from build123d import *

# Parameters (mm, degrees)
F0_R            = 56
F0_R_2          = 62.5
F1_DEPTH        = 35
F3_DEPTH        = 1
F4_W            = 26
F4_H            = 35
F5_DEPTH        = 50
F6_W            = 8
F6_H            = 10
F7_DEPTH        = 26
F8_R            = 17.5
F9_DEPTH        = 50
F10_R           = 2
F12_D           = 3
F12_DEPTH       = 8
F12_CBORE_D     = 5
F12_CBORE_DEPTH = 2
F14_D           = 3
F14_DEPTH       = 8
F14_CBORE_D     = 5
F14_CBORE_DEPTH = 2


with BuildPart() as f1:
    # F0 (on Top) → F1 (new body)
    with BuildSketch(Plane.XY):
        with Locations((-62.5, 0)):
            Circle(F0_R)
        with Locations((-62.5, 0)):
            Circle(F0_R_2)
        with Locations((-62.5, 0)):
            Circle(F0_R, mode=Mode.SUBTRACT)
    extrude(amount=F1_DEPTH)

    # F2 (on Right) → F3 (join)
    with BuildSketch(Plane.YZ):
        Polygon((-13, 0), (0, 0), (13, 0), (13, 35), (-13, 35), align=None)
    extrude(amount=-F3_DEPTH)

    # F4 (on face) → F5 (join)
    with BuildSketch(Plane.YZ):
        with Locations((0, 17.5)):
            Rectangle(F4_W, F4_H)
    extrude(amount=F5_DEPTH)

    # F6 (on face) → F7 (join)
    with BuildSketch(Plane.XZ.offset(13)):
        with Locations((42, 40)):
            Rectangle(F6_W, F6_H)
        with Locations((12, 40)):
            Rectangle(F6_W, F6_H)
    extrude(amount=-F7_DEPTH)

    # F8 (on face) → F9 (cut)
    with BuildSketch(Plane.XZ.offset(13)):
        with Locations((27, 21.5)):
            Circle(F8_R)
    extrude(amount=-F9_DEPTH, mode=Mode.SUBTRACT)

    # F10
    f10_edges = [f1.edges().sort_by_distance(p)[0] for p in [
        (46, 0, 35),
        (8, 0, 35),
    ]]
    fillet(f10_edges, radius=F10_R)

    # F12
    with Locations(Plane.YZ.offset(46)):
        with Locations((0, 41)):
            CounterBoreHole(F12_D / 2, F12_CBORE_D / 2, F12_CBORE_DEPTH, depth=F12_DEPTH)

    # F14
    with Locations(Plane(origin=(8, 0, 0), x_dir=(0, -1, 0), z_dir=(-1, 0, 0))):
        with Locations((0, 41)):
            CounterBoreHole(F14_D / 2, F14_CBORE_D / 2, F14_CBORE_DEPTH, depth=F14_DEPTH)


solid = f1.part
Geometry: final body of the model. Coordinates: model frame, mm. A direction names the side the tool comes from. Give positions to 0.01 mm unless a question says otherwise; leave off trailing zeros. Write each loop counter-clockwise with the first axis right and the second up, starting at its lowest first coordinate (ties: lowest second). Pieces come first, ordered by that corner, then holes.
(1) Cut plane C-C, the plane y = -25. Return loops of the section in (x, z), then the cut area to 3 significant figures.
(2) Access query for faces 1 (the flat face through (10, -2, 41)), 2 (the flat face through (16, 0, 39)), 3 (the flat face through (13, -13, 7)), 4 (the cylindrical face through (45.01, -0.54, 38.56)), 5 (the flat face through (-6, 0, 35)). Directions: +Z, -Z, +X, -X, +Y, -Y. A direction counts if a zero-diameter tool reaches every point of the face in a straight line with its end or side. Return the directions, or none.
(3) Ray query, line 1 (X direction, y = 2, z = 21); line 2 (Z direction, x = 45, y = 0); line 3 (X direction, y = 2.75, z = 21.5). Return the intervals inside material, ascending.
(4) Mould query, pull axis X, two halves, no side actions, for faces 6 (the flat face through (38, 0, 39)), 7 (the flat face through (44, 2, 41)), 8 (the cylindrical face through (8.99, 0.54, 38.56)). Classes: released by +X, released by -X, zero draft, split by the parting line, or undercut.
(5) Cut plane D-D, the plane x = 27. Return loops of the section in (y, z).
(6) Cut plane A-A, the plane x = -62.5. Return loops of the section in (y, z).
(7) First-contact query: P1, Ø10, axis at x = -63, z = 32.5, coming from the -Y side; P2, Ø1, axis at x = -46, z = 25, coming from the -Y side; P3, Ø1.8, axis at y = 0, z = 41, coming from the -X side; P4, Ø8, axis at y = 0, z = 41, coming from the +X side. Flat tips, straight axial feed; report the tip coordinate or a pass-through.
(8) Cut plane B-B, the plane z = 21.5. Return loops of the section in (x, y).
Values follow:
1. outline: (-119.78, 0) - (-112.61, 0) - (-112.61, 35) - (-119.78, 35) - close; (-12.39, 0) - (-5.22, 0) - (-5.22, 35) - (-12.39, 35) - close
1. area: 502 mm2
2. face 1: -X
2. face 2: +Z, +Y, -Y
2. face 3: +Z, -Z, +X, -Y
2. face 4: +X
2. face 5: +Z, -X, +Y, -Y
3. line 1: x = -124.97 to -118.46, -6.54 to 9.51, 44.49 to 50
3. line 2: z = 0 to 38.5, 43.5 to 45
3. line 3: x = -124.94 to -118.43, -6.57 to 9.5, 44.5 to 50
4. face 6: undercut
4. face 7: released by +X
4. face 8: zero draft
5. outline: (-13, 0) - (13, 0) - (13, 4) - (-13, 4) - close
6. outline: (-62.5, 0) - (-56, 0) - (-56, 35) - (-62.5, 35) - close; (56, 0) - (62.5, 0) - (62.5, 35) - (56, 35) - close
7. P1: stops at y = -62.5
7. P2: stops at y = -60.42
7. P3: passes through
7. P4: stops at x = 46
8. outline: (-1, -13) - (9.5, -13) - (9.5, 13) - (-1, 13) - (-1, 11.14) arc R62.5 ccw (long way) to (-1, -11.14) - close; (44.5, -13) - (50, -13) - (50, 13) - (44.5, 13) - close; hole circle Ø112 at (-62.5, 0)
